Here's how the part is built. I have some questions about the finished solid (model axes, mm). Face numbers are marked on the shaded views. A direction names the side the tool comes from. Give positions to 0.01 mm unless a question says otherwise; leave off trailing zeros. Write each loop counter-clockwise with the first axis right and the second up, starting at its lowest first coordinate (ties: lowest second). Pieces come first, ordered by that corner, then holes. Notation, with made-up numbers: (37, 36.5) - (70, 36.5) arc R11 ccw to (70, 51.5) - close; hole circle Ø9 at (52.25, 57.5). An arc over 180 degrees is marked (long way). Write each question's results on one line, items separated by ' | '. Start each with the question number.
Item 1: Suppose I cut it at A-A on x = 73. List the corners of the cut face in (y, z) for me, then the cut area to 3 significant figures.
Item 2: Will these pins go through, and if not, where does the flat tip stop? P1, Ø2, axis at x = 161, z = 15, coming from the -Y side; P2, Ø11, axis at x = 157, y = -1, coming from the +Z side; P3, Ø6, axis at x = 85.5, z = 10.5, coming from the -Y side; P4, Ø17.5, axis at y = 4, z = 7.5, coming from the -X side.
Item 3: Suppose I cut it at B-B on x = 159. List the corners of the cut face in (y, z) for me.
Item 4: Suppose I cut it at C-C on x = 214. List the corners of the cut face in (y, z) for me.
Item 5: Which directions (+Z, -Z, +X, -X, +Y, -Y) give clear straight access to the entire face, cutting with the end or side of a thin tool? Please do the marked faces 1 and 2.
Item 6: Please list where these lines run through material, in increasing order: line 1 along X through (y, z) = (18, -9); line 2 along Y through (x, z) = (170, -9); line 3 along Z through (x, y) = (146, 1).
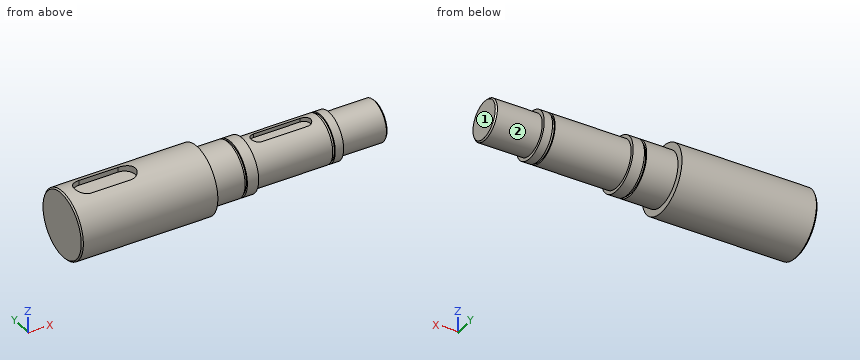
```python
from build123d import *

# Parameters (mm, degrees)
CHAMFER_1_SIZE      = 1
CUT_EXTRUDE_START   = -8
SKETCH_2_OUTSIDE_W  = 100.316
SKETCH_2_OUTSIDE_H  = 100.316
SKETCH_2_OUTSIDE_R  = 16.5
CUT_EXTRUDE_1_DEPTH = 1.85
CUT_EXTRUDE_START_2 = -10
SKETCH_3_OUTSIDE_W  = 100.316
SKETCH_3_OUTSIDE_H  = 100.316
SKETCH_3_OUTSIDE_R  = 18.75
CUT_EXTRUDE_2_DEPTH = 1.7
CUT_EXTRUDE_START_3 = 20
CUT_EXTRUDE_3_DEPTH = 214.689965553
CUT_EXTRUDE_START_4 = 14
CUT_EXTRUDE_4_DEPTH = 220.689965574


with BuildPart() as part:
    # 草图1 → 旋转1 (revolve)
    with BuildSketch(Plane.XY):
        Polygon((0, 0), (0, 25), (100, 25), (100, 20), (133, 20), (133, 17.5), (197, 17.5), (197, 15), (231, 15), (231, 0), align=None)
    revolve(axis=Axis((231, 0, 0), (-1, 0, 0)))

    # 倒角1
    chamfer_1_edges = [part.edges().sort_by_distance(p)[0] for p in [
        (0, -25, 0),
        (231, -15, 0),
    ]]
    chamfer(chamfer_1_edges, length=CHAMFER_1_SIZE)

    # 草图2 outside → 切除-拉伸1 (cut)
    with BuildSketch(Plane(origin=(197, 0, 0), x_dir=(0, 0, -1), z_dir=(1, 0, 0)).offset(CUT_EXTRUDE_START)):
        Rectangle(SKETCH_2_OUTSIDE_W, SKETCH_2_OUTSIDE_H)
        with Locations(Location((0, 0, 0), (0, 0, 90))):
            Circle(SKETCH_2_OUTSIDE_R, mode=Mode.SUBTRACT)
    extrude(amount=CUT_EXTRUDE_1_DEPTH, mode=Mode.SUBTRACT)

    # 草图3 outside → 切除-拉伸2 (cut)
    with BuildSketch(Plane(origin=(133, 0, 0), x_dir=(0, 0, -1), z_dir=(1, 0, 0)).offset(CUT_EXTRUDE_START_2)):
        Rectangle(SKETCH_3_OUTSIDE_W, SKETCH_3_OUTSIDE_H)
        with Locations(Location((0, 0, 0), (0, 0, 90))):
            Circle(SKETCH_3_OUTSIDE_R, mode=Mode.SUBTRACT)
    extrude(amount=CUT_EXTRUDE_2_DEPTH, mode=Mode.SUBTRACT)

    # 草图4 → 切除-拉伸3 (cut, through all)
    with BuildSketch(Plane.XY.offset(CUT_EXTRUDE_START_3)):
        with BuildLine():
            Line((17, 8), (46, 8))
            ThreePointArc((46, 8), (54, 0), (46, -8))
            Line((46, -8), (17, -8))
            ThreePointArc((17, -8), (9, 0), (17, 8))
        make_face()
    extrude(amount=CUT_EXTRUDE_3_DEPTH, mode=Mode.SUBTRACT)

    # 草图5 → 切除-拉伸4 (cut, through all)
    with BuildSketch(Plane.XY.offset(CUT_EXTRUDE_START_4)):
        with BuildLine():
            Line((144, 5), (178, 5))
            ThreePointArc((178, 5), (183, 0), (178, -5))
            Line((178, -5), (144, -5))
            ThreePointArc((144, -5), (139, 0), (144, 5))
        make_face()
    extrude(amount=CUT_EXTRUDE_4_DEPTH, mode=Mode.SUBTRACT)


solid = part.part
```
Checked values:
1) outline: circle Ø50 at (0, 0) | area: 1,960 mm^2
2) P1: stops at y = -10.5 | P2: stops at z = 16.77 | P3: stops at y = -23.85 | P4: stops at x = 0
3) outline: (-5, 14) - (-5, 16.77) arc R17.5 ccw (long way) to (5, 16.77) - (5, 14) - close
4) outline: circle Ø30 at (0, 0)
5) face 1: +Z, -Z, +X, +Y, -Y | face 2: +X
6) line 1: x = 0 to 100 | line 2: y = -15.01 to 15.01 | line 3: z = -17.47 to 14
